Verification items for the finished model (mm, model axes). Face numbers are marked on the shaded views. A direction names the side the tool comes from. Round coordinates to 2 decimals unless told otherwise and drop trailing zeros. Write each loop counter-clockwise with the first axis right and the second up, starting at its lowest first coordinate (ties: lowest second). Pieces come first, ordered by that corner, then holes. Notation, with made-up numbers: M -14,39.5 L 11,39.5 A22 cw 11,47.5 Z; hole C -32.5,-31 d5. An arc over 180 degrees is marked long. Answer in a Markdown table with one row per item. Add a question column.
1. Sectioned sample at B-B on z = 0. Record the cut outline in (x, y).
2. Sectioned sample at D-D on y = -2.25. Record the cut outline in (x, z).
3. Go/stop test with flat-tipped pins: pin 1 Ø1 at (x, y) = (-4, 1.5) entering from +Z; pin 2 Ø0.8 at (y, z) = (5, 2.5) entering from +X; pin 3 Ø0.6 at (y, z) = (4.5, -2) entering from -X. Record where each tip stops, or that it passes through.
4. Material ranges on probe 1 along Y at (x, z) = (1, 3); probe 2 along X at (y, z) = (-4, 0); probe 3 along X at (y, z) = (4.75, 0.5), recorded low to high.
5. Sectioned sample at C-C on y = 0. Record the cut outline in (x, z), plus the area to 3 significant figures.
6. Sectioned sample at A-A on x = 0. Record the cut outline in (y, z).
7. Set-up check for the marked faces 1 and 2: record each of +Z, -Z, +X, -X, +Y, -Y from which the full face is reachable in a straight line by a thin tool's end or side.
```python
from build123d import *

# Parameters (mm, degrees)
CROQUIS1_R                 = 4.5
SALIENTE_EXTRUIR1_DEPTH    = 4
CROQUIS2_R                 = 5
SALIENTE_EXTRUIR2_DEPTH    = 1
CROQUIS3_W                 = 0.5
CROQUIS3_H                 = 4.167915925
CORTAR_EXTRUIR1_DEPTH      = 6
CORTAR_EXTRUIR1_DEPTH_BACK = 6
CHAFL_N1_SIZE              = 0.5
CHAFL_N1_SIZE2             = 0.288675135
CROQUIS4_R                 = 4.5
SALIENTE_EXTRUIR3_DEPTH    = 1
CROQUIS5_R                 = 1.5
SALIENTE_EXTRUIR4_DEPTH    = 5


with BuildPart() as part:
    # Croquis1 → Saliente-Extruir1 (new body)
    with BuildSketch(Plane(origin=(0, 0, 0), x_dir=(1, 0, 0), z_dir=(0, 1, 0))):
        Circle(CROQUIS1_R)
    extrude(amount=SALIENTE_EXTRUIR1_DEPTH)

    # Croquis2 → Saliente-Extruir2 (add)
    with BuildSketch(Plane(origin=(0, 4, 0), x_dir=(1, 0, 0), z_dir=(0, 1, 0))):
        Circle(CROQUIS2_R)
    extrude(amount=SALIENTE_EXTRUIR2_DEPTH)

    # Croquis3 → Cortar-Extruir1 (cut, two sides)
    with BuildSketch(Plane.XY) as cortar_extruir1_sk:
        with Locations((0, 6.333957963)):
            Rectangle(CROQUIS3_W, CROQUIS3_H)
    extrude(amount=CORTAR_EXTRUIR1_DEPTH, mode=Mode.SUBTRACT)
    extrude(cortar_extruir1_sk.sketch, amount=-CORTAR_EXTRUIR1_DEPTH_BACK, mode=Mode.SUBTRACT)

    # Chaflán1
    chafl_n1_edges = [part.edges().sort_by_distance(p)[0] for p in [
        (-5, 5, 0),
        (3.622844187, 5, 3.446012188),
    ]]
    chafl_n1_side = [part.faces().sort_by_distance(p)[0] for p in [
        (-5, 4.5, 0),
    ]]
    chamfer(chafl_n1_edges, length=CHAFL_N1_SIZE, length2=CHAFL_N1_SIZE2, reference=chafl_n1_side[0])

    # Croquis4 → Saliente-Extruir3 (add)
    with BuildSketch(Plane.XZ):
        Circle(CROQUIS4_R)
    extrude(amount=SALIENTE_EXTRUIR3_DEPTH)

    # Croquis5 → Saliente-Extruir4 (add)
    with BuildSketch(Plane(origin=(0, -1, 0), x_dir=(-1, 0, 0), z_dir=(0, -1, 0))):
        Circle(CROQUIS5_R)
    extrude(amount=SALIENTE_EXTRUIR4_DEPTH)


solid = part.part
```
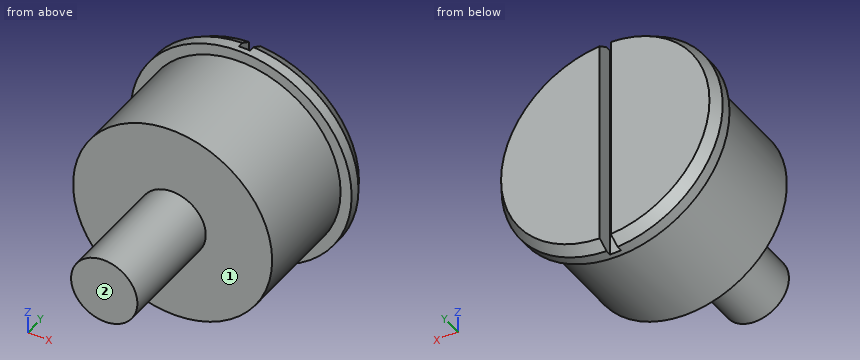
Geometry check:
| question | item | result |
|---|---|---|
| 1 | outline | M -5,4 L -4.5,4 L -4.5,-1 L -1.5,-1 L -1.5,-6 L 1.5,-6 L 1.5,-1 L 4.5,-1 L 4.5,4 L 5,4 L 5,4.5 L 4.71,5 L 0.25,5 L 0.25,4.25 L -0.25,4.25 L -0.25,5 L -4.71,5 L -5,4.5 Z |
| 2 | outline | C 0,0 d3 |
| 3 | pin 1 | stops at z = 2.83 |
| 3 | pin 2 | stops at x = 4.34 |
| 3 | pin 3 | stops at x = -4.7 |
| 4 | probe 1 | y = -1 to 5 |
| 4 | probe 2 | x = -1.5 to 1.5 |
| 4 | probe 3 | x = -4.83 to -0.25, 0.25 to 4.83 |
| 5 | outline | C 0,0 d9 |
| 5 | area | 63.6 mm2 |
| 6 | outline | M -6,-1.5 L -1,-1.5 L -1,-4.5 L 4,-4.5 L 4,-5 L 4.25,-5 L 4.25,5 L 4,5 L 4,4.5 L -1,4.5 L -1,1.5 L -6,1.5 Z |
| 7 | face 1 | -Y |
| 7 | face 2 | +Z, -Z, +X, -X, -Y |
